Drawing for the job (mm, zero at the part's lowest x, y, z). Coordinates: 2 decimals unless noted, no trailing zeros. Write each loop counter-clockwise with the first axis right and the second up, starting at its lowest first coordinate (ties: lowest second). Pieces come first, ordered by that corner, then holes. Notation, with made-up numbers: M -32,55.25 L 17,55.25 A24 ccw 17,82.25 Z; hole C 85.25,35 d3. An arc over 180 degrees is marked long. Use a Markdown table: item, result. Add a question column.
Q1. Slice it at C-C on x = 11.25. Write the cut outline in (y, z).
Q2. Slice it at A-A on y = 2.5. Write the cut outline in (x, z), then the cut area to 3 significant figures.
Q3. Slice it at D-D on y = 9. Write the cut outline in (x, z), then the cut area to 3 significant figures.
Q4. Wall check: L1, parallel to X at y = 4, z = 0.45; L2, parallel to Y at x = 3.25, z = 0.5; L3, parallel to X at y = 9.25, z = 0.3. Give the ranges that are in metal, low to high. Write a range as from..to.
Q5. Slice it at B-B on z = 0.4. Write the cut outline in (x, y).
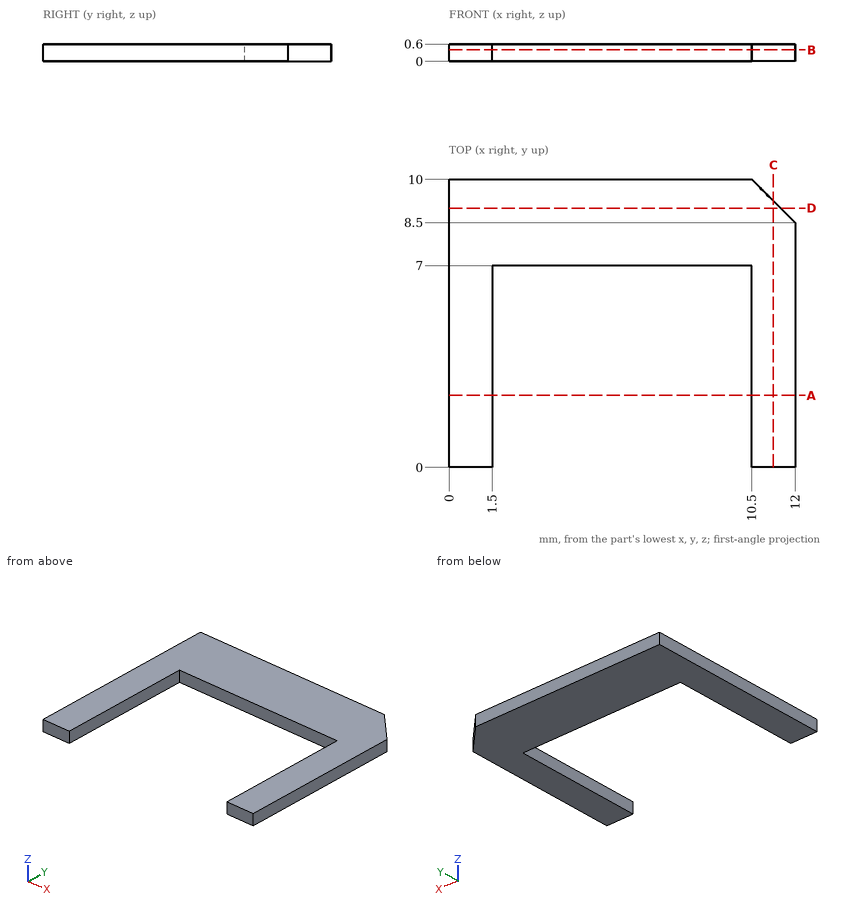
Recorded:
| question | item | result |
|---|---|---|
| 1 | outline | M 0,0 L 9.25,0 L 9.25,0.6 L 0,0.6 Z |
| 2 | outline | M 0,0 L 1.5,0 L 1.5,0.6 L 0,0.6 Z; M 10.5,0 L 12,0 L 12,0.6 L 10.5,0.6 Z |
| 2 | area | 1.80 mm² |
| 3 | outline | M 0,0 L 11.5,0 L 11.5,0.6 L 0,0.6 Z |
| 3 | area | 6.90 mm² |
| 4 | L1 | 0..1.5, 10.5..12 |
| 4 | L2 | 7..10 |
| 4 | L3 | 0..11.25 |
| 5 | outline | M 0,0 L 1.5,0 L 1.5,7 L 10.5,7 L 10.5,0 L 12,0 L 12,8.5 L 10.5,10 L 0,10 Z |
